The figure shows three views and two pictorial views of one solid part (mm, origin at its lowest corner). Answer the questions. A direction names the side the tool comes from. Round coordinates to 2 decimals unless told otherwise and drop trailing zeros. Order: outer loops, then holes, each group sorted by start corner. A loop starts at its lowest first (then second) coordinate and runs counter-clockwise, first axis right, second up.
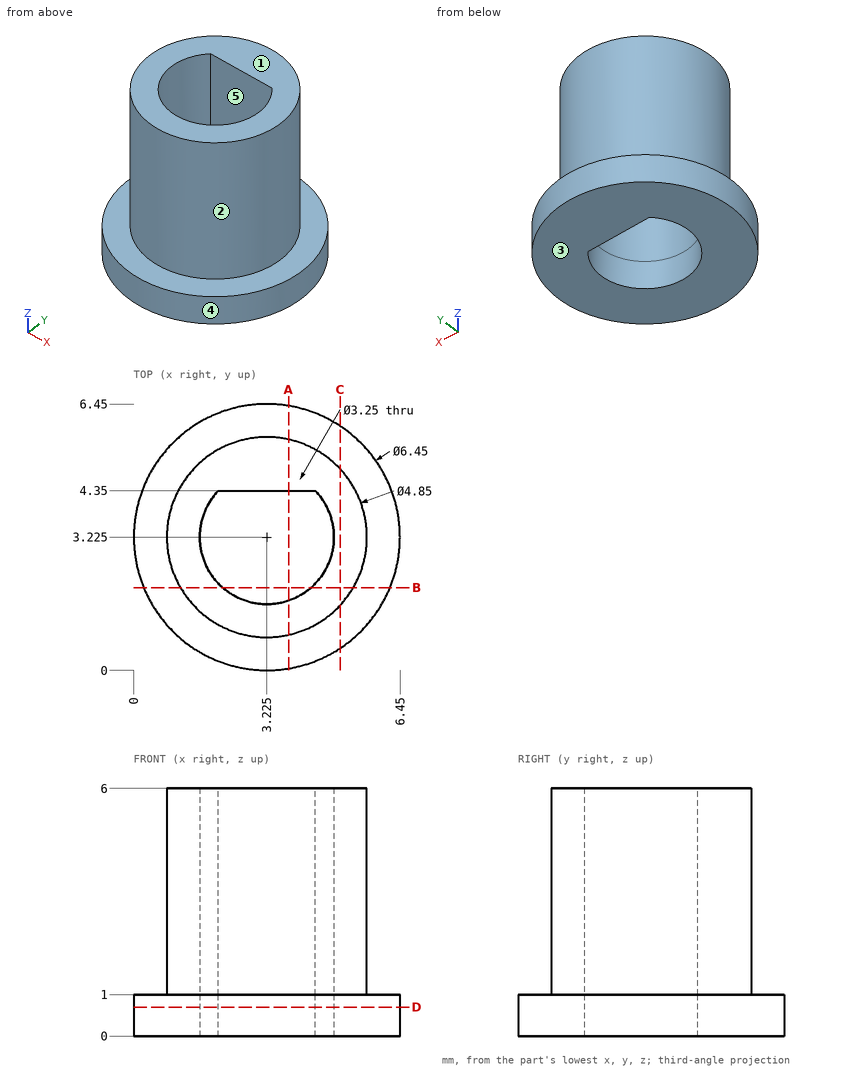
Item 1: Find section C-C (x = 5). Write down the section's boundary in (y, z).
Item 2: For a pull along X with two mould halves and no side action, classify the marked faces 3, 4 and 5 as released by +X, released by -X, zero draft, split by the parting line, or undercut.
Item 3: Given pin 1 (3 mm diameter, centred on x = 6, y = 5.5, fed in from +Z); pin 2 (0.7 mm diameter, centred on x = 3.5, z = 4.5, fed in from -Y); pin 3 (1.5 mm diameter, centred on y = 1.5, z = 2, fed in from +X); pin 4 (2 mm diameter, centred on x = 3.225, y = 3.225, fed in from +Z), each flat-ended and moving along its own axis, determine where each tip first touches the part or whether it passes through.
Item 4: Find section B-B (y = 2). Write down the section's boundary in (x, z).
Item 5: Find the intervals of material crossed by line 1 along Y through (x, z) = (3.25, 5.3); line 2 along Z through (x, y) = (0.75, 4.25); line 3 along X through (y, z) = (2.75, 1.3), in increasing order.
Item 6: Find section A-A (x = 3.75). Write down the section's boundary in (y, z), plus the area to 3 significant figures.
Item 7: A tool of negligible diameter and unlimited length cuts with its end or side. For the marked faces 1 and 2, from which of +Z, -Z, +X, -X, +Y, -Y can it reach the whole face along a straight path? Write none if from no direction.
Item 8: Find section D-D (z = 0.7). Write down the section's boundary in (x, y) (3 decimals), plus the area to 3 significant figures.
Model answer:
1. outline: (0.53, 0) - (5.92, 0) - (5.92, 1) - (4.88, 1) - (4.88, 6) - (1.57, 6) - (1.57, 1) - (0.53, 1) - close
2. face 3: zero draft
2. face 4: split by the parting line
2. face 5: undercut
3. pin 1: stops at z = 6
3. pin 2: stops at y = 0.8
3. pin 3: stops at x = 5.45
3. pin 4: passes through
4. outline: (0.24, 0) - (2.16, 0) - (2.16, 6) - (1.13, 6) - (1.13, 1) - (0.24, 1) - close; (4.29, 0) - (6.21, 0) - (6.21, 1) - (5.32, 1) - (5.32, 6) - (4.29, 6) - close
5. line 1: y = 0.8 to 1.6, 4.35 to 5.65
5. line 2: z = 0 to 1
5. line 3: x = 0.85 to 1.67, 4.78 to 5.6
6. outline: (0.04, 0) - (1.69, 0) - (1.69, 6) - (0.86, 6) - (0.86, 1) - (0.04, 1) - close; (4.35, 0) - (6.41, 0) - (6.41, 1) - (5.59, 1) - (5.59, 6) - (4.35, 6) - close
6. area: 14.1 mm2
7. face 1: +Z, +X, -X, +Y, -Y
7. face 2: +Z
8. outline: circle Ø6.45 at (3.225, 3.225); hole (2.052, 4.35) arc R1.625 ccw (long way) to (4.398, 4.35) - close
8. area: 25.2 mm2
